from build123d import *

# Parameters (mm, degrees)
F1_DEPTH = 30
F3_D     = 17


with BuildPart() as f1:
    # F0 (on Right) → F1 (new body)
    with BuildSketch(Plane.YZ):
        Polygon((46.7509815469, 15.6090386026), (46.7509815469, 50.6090386026), (21.7509815469, 50.6090386026), (21.7509815469, 35.6090386026), (-3.2490184531, 35.6090386026), (-3.2490184531, 15.6090386026), align=None)
    extrude(amount=F1_DEPTH)

    # F3 (through all)
    with Locations(Plane(origin=(0, 0, 0), x_dir=(1, 0, 0), z_dir=(0, 0, -1))):
        with Locations((15, -9.2509815469)):
            Hole(F3_D / 2)


solid = f1.part
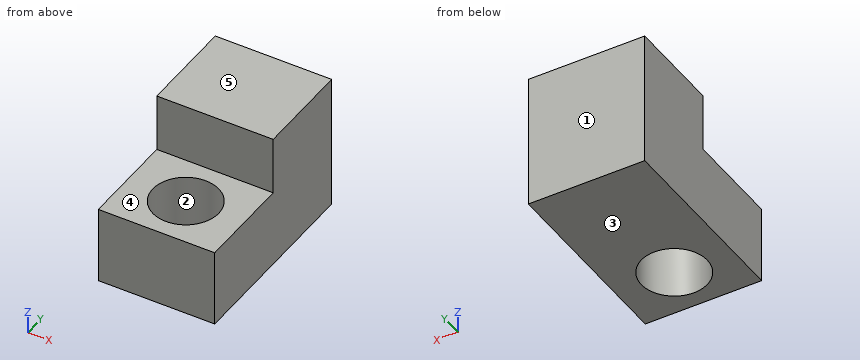
The model under review builds one solid part; all positions refer to its coordinate system, in mm. Face numbers are marked on the shaded views. A direction names the side the tool comes from. Round coordinates to 2 decimals unless told otherwise and drop trailing zeros. Loops run counter-clockwise (first coordinate to the right, second up) from the corner with the lowest first, then second, coordinate; pieces in that order, holes last. Notation, with made-up numbers: (13.25, 23.25) -> (54.25, 23.25) arc R29 cw to (54.25, 51.25) -> close; hole circle Ø3 at (44, 81). An arc over 180 degrees is marked (long way). One line per question, with ' | ' between items. Start each with the question number.
Item 1: Add section B-B, the plane y = 17. Write out the cut boundary in (x, z).
Item 2: Machinability: for the marked faces 4 and 5, which of the approach directions +Z, -Z, +X, -X, +Y, -Y give a long, thin tool a straight path to every point of the face, cutting with its end or side? Answer none if there is none.
Item 3: Add section C-C, the plane y = 7. Write out the cut boundary in (x, z), then the cut area to 3 significant figures.
Item 4: Add section D-D, the plane x = 25.5. Write out the cut boundary in (y, z), then the cut area to 4 significant figures.
Item 5: For pin 1 (16.5 mm diameter, centred on x = 14, z = 44, fed in from -Y), flat-tipped, find the tip position at first contact; note if it passes through.
Item 6: Wall thickness on line 1 along Y through (x, z) = (15, 28); line 2 along Y through (x, z) = (20.5, 47); line 3 along Z through (x, y) = (22.25, 4): over which ranges is each line inside the solid? List them lowest first. Write a range as [from, to].
Item 7: Draft analysis for pull direction Y (two halves, no side actions). For the marked faces 1, 2 and 3, state which applies: +Y half, -Y half, draft (parallel to the pull), parting line (faces both ways), or undercut.
Item 8: Add section A-A, the plane x = 15. Write out the cut boundary in (y, z), then the cut area to 4 significant figures.
Return value:
1) outline: (0, 15.61) -> (11.51, 15.61) -> (11.51, 35.61) -> (0, 35.61) -> close; (18.49, 15.61) -> (30, 15.61) -> (30, 35.61) -> (18.49, 35.61) -> close
2) face 4: +Z, +X, -X, -Y | face 5: +Z, +X, -X, +Y, -Y
3) outline: (0, 15.61) -> (6.8, 15.61) -> (6.8, 35.61) -> (0, 35.61) -> close; (23.2, 15.61) -> (30, 15.61) -> (30, 35.61) -> (23.2, 35.61) -> close | area: 272 mm2
4) outline: (-3.25, 15.61) -> (46.75, 15.61) -> (46.75, 50.61) -> (21.75, 50.61) -> (21.75, 35.61) -> (-3.25, 35.61) -> close | area: 1,375 mm2
5) pin 1: stops at y = 21.75
6) line 1: y = [-3.25, 0.75], [17.75, 46.75] | line 2: y = [21.75, 46.75] | line 3: z = [15.61, 35.61]
7) face 1: +Y half | face 2: undercut | face 3: draft
8) outline: (-3.25, 15.61) -> (0.75, 15.61) -> (0.75, 35.61) -> (-3.25, 35.61) -> close; (17.75, 15.61) -> (46.75, 15.61) -> (46.75, 50.61) -> (21.75, 50.61) -> (21.75, 35.61) -> (17.75, 35.61) -> close | area: 1,035 mm2
